Design review of the part built by this model. Coordinates are the model's own, in mm. Round coordinates to 2 decimals unless told otherwise and drop trailing zeros. Loops run counter-clockwise (first coordinate to the right, second up) from the corner with the lowest first, then second, coordinate; pieces in that order, holes last. Notation, with made-up numbers: (77.5, -8) - (116.5, -8) arc R26 ccw to (116.5, 8) - close; hole circle Ø3 at (5, 69.25). An arc over 180 degrees is marked (long way). One line per question, with ' | ' between items. Start each with the question number.
from build123d import *

# Parameters (mm, degrees)
SKETCH_1_R          = 12.5
SKETCH_1_R_2        = 11.5
EXTRUDE_1_DEPTH     = 820
SKETCH_2_R          = 2.5
CUT_EXTRUDE_1_DEPTH = 821.190526646


with BuildPart() as part:
    # Эскиз1 → Вытянуть-Тонкостенный1 (new body)
    with BuildSketch(Plane(origin=(0, 0, 0), x_dir=(1, 0, 0), z_dir=(0, 1, 0))):
        Circle(SKETCH_1_R)
        Circle(SKETCH_1_R_2, mode=Mode.SUBTRACT)
    extrude(amount=EXTRUDE_1_DEPTH)

    # Эскиз2 → Вырез-Вытянуть1 (cut, symmetric)
    with BuildSketch(Plane(origin=(0, 0, 0), x_dir=(0, 0, -1), z_dir=(1, 0, 0))):
        with Locations((0, 110)):
            Circle(SKETCH_2_R)
        with Locations((0, 20)):
            Circle(SKETCH_2_R)
    cut_extrude_1 = extrude(amount=CUT_EXTRUDE_1_DEPTH, both=True, mode=Mode.SUBTRACT)

    # Зеркальное отражение1: Вырез-Вытянуть1 across plane
    add(cut_extrude_1.mirror(Plane(origin=(0, 410, 0), x_dir=(0, 0, 1), z_dir=(0, -1, 0))), mode=Mode.SUBTRACT)


solid = part.part
1. Take a section at A-A, the plane x = 0. Give the boundary of the cut face in (y, z).
2. To check wall thickness, follow line 1 along Y through (x, z) = (11.85, 0); line 2 along X through (y, z) = (588, -1.25); line 3 along Z through (x, y) = (0, 111.5). State the ranges of each line that lie inside material, in increasing order.
3. Clearance check with flat-ended pins moving along their axes: P1, Ø3, axis at y = 800, z = 0, coming from the +X side; P2, Ø8, axis at y = 710, z = 0, coming from the +X side; P3, Ø1.5, axis at x = -4.5, y = 178, coming from the -Z side; P4, Ø4, axis at x = -3, y = 493, coming from the -Z side. State where each tip first meets the part, or that it passes through.
4. The part is to be moulded in two halves that separate along Z. For faces 1 (the face through (11, 0, 4)), 2 (the face through (11.923, 404.26, -3.755)), 3 (the face through (-1.5, 404.3, -11.4)), say which applies: pulls with the +Z half, pulls with the -Z half, needs draft (parallel to the pull), parting line crosses it, or undercut.
5. Take a section at B-B, the plane y = 133.5. Give the boundary of the cut face in (x, z).
Answer list:
1) outline: (0, -12.5) - (820, -12.5) - (820, -11.5) - (0, -11.5) - close; (0, 11.5) - (820, 11.5) - (820, 12.5) - (0, 12.5) - close
2) line 1: y = 0 to 17.5, 22.5 to 107.5, 112.5 to 707.5, 712.5 to 797.5, 802.5 to 820 | line 2: x = -12.44 to -11.43, 11.43 to 12.44 | line 3: z = -12.5 to -11.5, 11.5 to 12.5
3) P1: passes through | P2: stops at x = 12.5 | P3: stops at z = -11.92 | P4: stops at z = -12.46
4) face 1: needs draft | face 2: parting line crosses it | face 3: undercut
5) outline: circle Ø25 at (0, 0); hole circle Ø23 at (0, 0)
